from build123d import *

# Parameters (mm, degrees)
F1_DEPTH = 50.8
F2_R     = 11.859009
F4_DEPTH = 50.8
F5_DEPTH = 76.2


with BuildPart() as f1:
    # F0 (on Front) → F1 (new body)
    with BuildSketch(Plane.XZ):
        Polygon((0, 63.13429), (0, 0), (304.8, 0), (304.8, 17.081553), align=None)
    extrude(amount=F1_DEPTH)

    # F2 (on face) → F4 (cut)
    with BuildSketch(Plane(origin=(0, 0, 0), x_dir=(0, -1, 0), z_dir=(-1, 0, 0))):
        with Locations((25.4, 25.630444)):
            Circle(F2_R)
    extrude(amount=-F4_DEPTH, mode=Mode.SUBTRACT)

    # F3 (on face) → F5 (cut)
    with BuildSketch(Plane.XZ.offset(50.8)):
        Polygon((0, 63.13429), (0, 40.274497), (19.827113, 51.353723), (53.36424, 51.353723), (96.555851, 30.648993), (152.476817, 17.081553), (239.942938, 13.801008), (247.112304, 17.027218), (247.112304, 6.990121), (0, 10.574799), (0, 0), (304.8, 0), (304.8, 17.081553), align=None)
    extrude(amount=-F5_DEPTH, mode=Mode.SUBTRACT)


solid = f1.part
Here's how the part is built. I have some questions about the finished solid (model axes, mm). A direction names the side the tool comes from. Round coordinates to 2 decimals unless told otherwise and drop trailing zeros. Order: outer loops, then holes, each group sorted by start corner. A loop starts at its lowest first (then second) coordinate and runs counter-clockwise, first axis right, second up. Notation, with made-up numbers: M 72,87 L 128,87 A8 ccw 128,101 Z; hole C 77.25,84.5 d7. An arc over 180 degrees is marked long. Return JSON: item names as keys, results as strings. Group by question number.
1. I'm going to push flat-ended pins straight in: pin 1 Ø8 at (x, y) = (169.5, -17.5) entering from -Z; pin 2 Ø1 at (y, z) = (-26, 24) entering from -X; pin 3 Ø2 at (y, z) = (-22, 36.5) entering from +X. Where does each tip first touch, or does it pass through?
2. If we section it at C-C on z = 34: List the corners of the cut face in (x, y) for me, then the cut area to 3 significant figures.
3. On a 3-axis mill with a long thin cutter (end or side, diameter ignored), from which of +Z, -Z, +X, -X, +Y, -Y can I reach the whole of each face in a straight line? I mean faces 4 (the face through (50.8, -25, 26)), 5 (the face through (243.5, -25.8, 15.4)), 6 (the face through (124.12, -25.76, 23.96)). Say none if no direction works.
4. If we section it at D-D on y = -11: List the corners of the cut face in (x, z) for me.
5. If we mould it in two halves opening along Z, with no side actions, what happens to faces 1 (the face through (25.044, -36.711, 29.193)), 2 (the face through (0, -13.8, 28.9)), 3 (the face through (36, -26, 51.354))? For each: pulls with the +Z half, pulls with the -Z half, needs draft (parallel to the pull), parting line crosses it, or undercut.
6. If we section it at B-B on x = 24: List the corners of the cut face in (y, z) for me, then the cut area to 3 significant figures.
7. Please list where these lines run through material, in increasing order: probe 1 along Z at (x, y) = (24, -25.4); probe 2 along X at (y, z) = (-14.5, 33.5); probe 3 along Z at (x, y) = (33.5, -25.4).
8. If we section it at A-A on y = -25.4: List the corners of the cut face in (x, z) for me.
Reply:
{
 "1": {"pin 1": "z = 8.06", "pin 2": "x = 50.8", "pin 3": "x = 86.44"},
 "2": {"outline": "M 0,-50.8 L 89.57,-50.8 L 89.57,0 L 0,0 L 0,-17 L 50.8,-17 L 50.8,-33.8 L 0,-33.8 Z", "area": "3,700 mm^2"},
 "3": {"face 4": "-X", "face 5": "+Z, +Y, -Y", "face 6": "+Z, +X, +Y, -Y"},
 "4": {"outline": "M 0,10.57 L 247.11,6.99 L 247.11,17.03 L 239.94,13.8 L 152.48,17.08 L 96.56,30.65 L 53.36,51.35 L 19.83,51.35 L 0,40.27 Z"},
 "5": {"face 1": "undercut", "face 2": "needs draft", "face 3": "pulls with the +Z half"},
 "6": {"outline": "M -50.8,10.23 L 0,10.23 L 0,51.35 L -50.8,51.35 Z; hole C -25.4,25.63 d23.72", "area": "1,650 mm^2"},
 "7": {"probe 1": "10.23 to 13.77, 37.49 to 51.35", "probe 2": "0 to 90.61", "probe 3": "10.09 to 13.77, 37.49 to 51.35"},
 "8": {"outline": "M 0,10.57 L 247.11,6.99 L 247.11,17.03 L 239.94,13.8 L 152.48,17.08 L 96.56,30.65 L 53.36,51.35 L 19.83,51.35 L 0,40.27 L 0,37.49 L 50.8,37.49 L 50.8,13.77 L 0,13.77 Z"}
}
